Part print with two shaded views. Sizes in mm from the minimum x, y, z corner. A direction names the side the tool comes from. Round coordinates to 2 decimals unless told otherwise and drop trailing zeros. Write each loop counter-clockwise with the first axis right and the second up, starting at its lowest first coordinate (ties: lowest second). Pieces come first, ordered by that corner, then holes. Notation, with made-up numbers: M -12.75,-20.75 L 25.25,-20.75 A28 ccw 25.25,4.25 Z; hole C -25,-33 d9. An arc over 180 degrees is marked long. Use one line per item in the form item = value. Start each with the question number.
Item 1: Flat gauge pins, fed straight in: pin 1 Ø4 at (y, z) = (17.5, 85.5) entering from -X; pin 2 Ø1 at (x, y) = (25, 27.5) entering from -Z; pin 3 Ø4 at (y, z) = (13.5, 64.5) entering from +X; pin 4 Ø8 at (x, y) = (32, 22) entering from -Z. Where does each tip first touch, or does it go through?
Item 2: Probe L1, parallel to Z at x = 16.5, y = 54; L2, parallel to Z at x = 44, y = 52.5; L3, parallel to Y at x = 30, z = 121. List the from-to ranges inside material, lowest first.
Item 3: Cut at D-D, the plane y = 38. Give the cut face in (x, z).
Item 4: Mould opens along Z. For the marked faces 1, 2, 3 and 4 say: +Z half, -Z half, draft (parallel to the pull), parting line (faces both ways), or undercut.
Item 5: Cut at A-A, the plane x = 30. Give the cut face in (y, z), then the cut area to 4 significant figures.
Item 6: Cut at C-C, the plane z = 88.5. Give the cut face in (x, y), then the cut area to 3 significant figures.
Item 7: Which spindle directions (+Z, -Z, +X, -X, +Y, -Y) get a long thin tool onto all of the face, cutting with end or side? Do the marked faces 5, 6 and 7. Say none if no direction does.
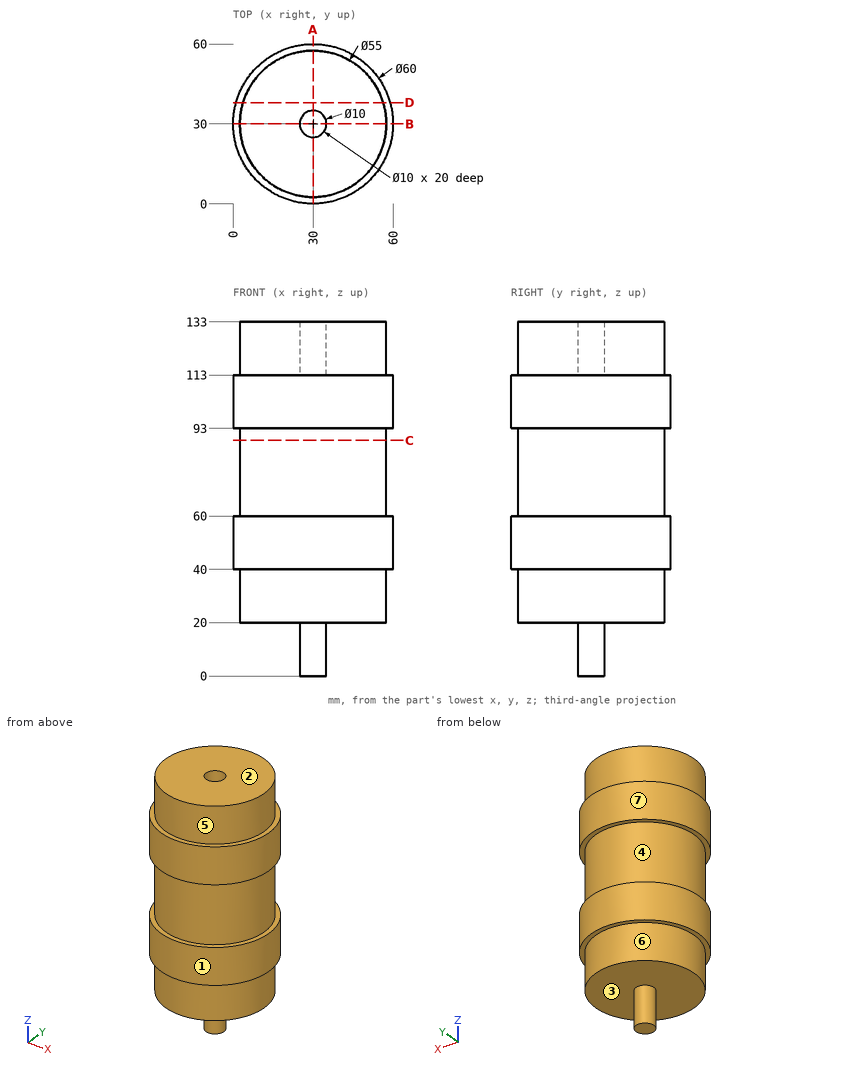
Model answer:
q1.pin_1 = 4.58
q1.pin_2 = 20
q1.pin_3 = 53.37
q1.pin_4 = 0
q2.L1 = 40 to 60, 93 to 113
q2.L2 = 20 to 133
q2.L3 = 2.5 to 25, 35 to 57.5
q3.outline = M 1.09,40 L 3.69,40 L 3.69,20 L 56.31,20 L 56.31,40 L 58.91,40 L 58.91,60 L 56.31,60 L 56.31,93 L 58.91,93 L 58.91,113 L 56.31,113 L 56.31,133 L 3.69,133 L 3.69,113 L 1.09,113 L 1.09,93 L 3.69,93 L 3.69,60 L 1.09,60 Z
q4.face_1 = draft
q4.face_2 = +Z half
q4.face_3 = -Z half
q4.face_4 = undercut
q5.outline = M 0,40 L 2.5,40 L 2.5,20 L 25,20 L 25,0 L 35,0 L 35,20 L 57.5,20 L 57.5,40 L 60,40 L 60,60 L 57.5,60 L 57.5,93 L 60,93 L 60,113 L 57.5,113 L 57.5,133 L 35,133 L 35,113 L 25,113 L 25,133 L 2.5,133 L 2.5,113 L 0,113 L 0,93 L 2.5,93 L 2.5,60 L 0,60 Z
q5.area = 6,415 mm²
q6.outline = C 30,30 d55
q6.area = 2,380 mm²
q7.face_5 = +Z
q7.face_6 = -Z
q7.face_7 = +Z, -Z
